Autodesk Inventor part; units mm, degrees
ref_plane "YZ Plane" through (0, 0, 0) normal (1, 0, 0) x (0, 1, 0)
ref_plane "XZ Plane" through (0, 0, 0) normal (0, 1, 0) x (-1, 0, 0)
ref_plane "XY Plane" through (0, 0, 0) normal (0, 0, 1) x (1, 0, 0)
sketch "Sketch1" plane through (0, 0, 0) normal (0, 1, 0) x (-1, 0, 0)
  line L0 (0, 0) -> (25.4, 0)
  line L1 (25.4, 0) -> (25.4, -127)
  line L2 (25.4, -127) -> (0, -127)
  line L3 (0, -127) -> (0, 0)
  line L4 (30.48, 5.08) -> (-5.08, 5.08)
  line L5 (-5.08, 5.08) -> (-5.08, -132.08)
  line L6 (-5.08, -132.08) -> (30.48, -132.08)
  line L7 (30.48, -132.08) -> (30.48, 5.08)
  dimension "d0" = 25.4
  dimension "d1" = 127
  dimension "d2" = 5.08
  dimension "d3" = 5.08
  dimension "d4" = 5.08
  dimension "d5" = 5.08
extrude "Extrusion1" add sketch "Sketch1" along normal blind 38.1
sketch "Sketch2" plane through (0, 38.1, 0) normal (0, 1, 0) x (1, 0, 0)
  line L0 (-30.48, -5.08) -> (5.08, -5.08)
  line L1 (5.08, -5.08) -> (-62.5812, -5.08)
  line L2 (-62.5812, -5.08) -> (-62.5812, 0)
  line L3 (-62.5812, 0) -> (0, 0)
  line L4 (-25.4, 127) -> (0, 127)
  line L5 (0, 127) -> (-62.5812, 127)
  line L6 (5.08, -5.08) -> (5.08, 132.08)
  line L7 (5.08, -5.08) -> (-62.5812, -5.08)
  line L8 (-62.5812, 132.08) -> (5.08, 132.08)
  line L9 (5.08, 132.08) -> (5.08, -5.08)
  line L10 (-62.5812, 132.08) -> (-47.0844, 132.08)
  line L11 (-62.5812, 127) -> (-62.5812, 132.08)
  line L12 (0, 127) -> (0, 0)
  line L13 (0, 0) -> (0, 127)
  line L14 (0, 127) -> (-62.5812, 127)
  line L15 (-62.5812, 132.08) -> (3.2473, 132.08)
  line L16 (5.08, 132.08) -> (-30.48, 132.08)
extrude "Extrusion2" add sketch "Sketch2" along normal blind 25.4
sketch "Sketch5" plane through (0, 38.1, 0) normal (0, -1, 0) x (1, 0, 0)
  line L0 (-62.5812, -132.08) -> (-62.5812, -127)
  line L1 (-30.48, -132.08) -> (-30.48, 5.08)
  line L2 (-62.5812, -132.08) -> (-30.48, -132.08)
  line L3 (-30.48, -132.08) -> (-30.48, -126.7104)
  line L4 (-30.48, -126.7104) -> (-62.5812, -126.7104)
  line L5 (-62.5812, -126.7104) -> (-62.5812, -132.08)
  line L6 (-62.5812, 0) -> (-62.5812, 5.08)
  line L7 (-30.48, 5.08) -> (5.08, 5.08)
  line L8 (-62.5812, 0) -> (-30.48, 0)
  line L9 (-30.48, 0) -> (-30.48, 5.08)
  line L10 (-30.48, 5.08) -> (-62.5812, 5.08)
  line L11 (-62.5812, 5.08) -> (-62.5812, 0)
  point P0 (0, 0)
extrude "Extrusion3" add sketch "Sketch5" along normal blind 38.1
sketch "Sketch6" plane through (-30.48, 0, 0) normal (-1, 0, 0) x (0, 0, 1)
  line L0 (-25.4, 7.62) -> (-38.1, 7.62)
  line L1 (-38.1, 7.62) -> (-38.1, 29.972)
  line L2 (-38.1, 29.972) -> (-25.4, 29.972)
  line L3 (-25.4, 29.972) -> (-25.4, 7.62)
  line L4 (-126.7104, 0) -> (0, 0)
  line L5 (0, 63.5) -> (0, 0)
  line L6 (-88.6104, 7.62) -> (-101.3104, 7.62)
  line L7 (-101.3104, 7.62) -> (-101.3104, 29.972)
  line L8 (-101.3104, 29.972) -> (-88.6104, 29.972)
  line L9 (-88.6104, 29.972) -> (-88.6104, 7.62)
  line L10 (-126.7104, 38.1) -> (-126.7104, 0)
  point P0 (-25.4, 18.796)
  point P1 (-88.6104, 18.796)
  point P2 (-126.7104, 19.05)
  point P3 (-101.3104, 18.796)
  dimension "d12" = 12.7
  dimension "d13" = 22.352
  dimension "d14" = 7.62
  dimension "d15" = 25.4
  dimension "d16" = 12.7
  dimension "d17" = 22.352
  dimension "d18" = 25.4
  dimension "d19" = 7.62
extrude "Extrusion4" cut sketch "Sketch6" against normal blind 12.7
sketch "Sketch7" plane through (0, 0, -127) normal (-1, 0, 0) x (0, 0, 1)
  line L0 (51.0896, 34.798) -> (38.3896, 34.798)
  line L1 (38.3896, 34.798) -> (38.3896, 57.15)
  line L2 (38.3896, 57.15) -> (51.0896, 57.15)
  line L3 (51.0896, 57.15) -> (51.0896, 34.798)
  line L4 (38.3896, 29.972) -> (38.3896, 7.62)
  line L5 (0, 63.5) -> (127, 63.5)
  line L6 (114.3, 34.798) -> (101.6, 34.798)
  line L7 (101.6, 34.798) -> (101.6, 57.15)
  line L8 (101.6, 57.15) -> (114.3, 57.15)
  line L9 (114.3, 57.15) -> (114.3, 34.798)
  line L10 (101.6, 31.5595) -> (101.6, 9.2075)
  line L11 (101.6, 29.972) -> (101.6, 7.62)
  point P0 (127, 0)
  point P1 (51.0896, 45.974)
  point P2 (38.3896, 18.796)
  point P3 (44.7396, 57.15)
  point P4 (114.3, 45.974)
  point P5 (101.6, 20.3835)
  point P6 (107.95, 57.15)
  dimension "d22" = 12.7
  dimension "d23" = 22.352
  dimension "d24" = 0
  dimension "d25" = 6.35
  dimension "d26" = 12.7
  dimension "d27" = 22.352
  dimension "d28" = 0
  dimension "d29" = 6.35
extrude "Extrusion5" cut sketch "Sketch7" against normal blind 12.7
properties part number "Base1"
Geometry check sheet. Reference: the model listing, model coordinates, mm. A direction names the side the tool comes from. Coordinates: 2 decimals unless noted, no trailing zeros. Order: outer loops, then holes, each group sorted by start corner. A loop starts at its lowest first (then second) coordinate and runs counter-clockwise, first axis right, second up. Notation, with made-up numbers: (-26.5, -37) - (4.5, -37) arc R12 cw to (4.5, -32) - close; hole circle Ø7 at (-31.75, 55.25). An arc over 180 degrees is marked (long way). Answer as a JSON object with one key per item and string values. Group by question number.
Item 1: Sectioned sample at C-C, the plane z = -86. Record the cut outline in (x, y), and give its area (3 significant figures).
Item 2: Draft check along Z on faces 1 (the face through (-29, 31, 5.08)), 2 (the face through (3, 57.15, -82)), 3 (the face through (5.08, 31, -63)). Enter one of: +Z half, -Z half, draft (parallel to the pull), parting line (faces both ways), or undercut.
Item 3: Scan lines: probe 1 along Z at (x, y) = (-8.5, 53.5); probe 2 along Z at (x, y) = (-58.5, 6); probe 3 along X at (y, z) = (6.5, -35). Record each from-to range of solid material in increasing order.
Item 4: Sectioned sample at B-B, the plane x = -5. Record the cut outline in (y, z).
Item 5: Sectioned sample at A-A, the plane y = 39.5. Record the cut outline in (x, z).
Item 6: Sectioned sample at D-D, the plane y = 13. Record the cut outline in (x, z), and give its area (3 significant figures).
Item 7: Depth check by flat-ended pin: pin 1 Ø19 at (y, z) = (21.5, -47.5) entering from -X; pin 2 Ø3 at (y, z) = (40.5, -12) entering from -X; pin 3 Ø2.5 at (x, z) = (-28.5, -96) entering from +Y. Enter the tip coordinate at first touch or a pass-through.
Item 8: Tool access check on faces 4 (the face through (-30.48, 19, -64)), 5 (the face through (3, 34.798, -19)), 6 (the face through (-28, 7.62, -32)), 7 (the face through (3, 57.15, -19)), 8 (the face through (-25.4, 19, -63)). Record the directions out of +Z, -Z, +X, -X, +Y, -Y that give a thin tool (end or side, any length) a straight path to the whole face; none if there is none.
Resolved:
{
 "1": {"outline": "(-30.48, 0) - (-25.4, 0) - (-25.4, 38.1) - (-30.48, 38.1) - close; (0, 0) - (5.08, 0) - (5.08, 34.8) - (0, 34.8) - close; (0, 57.15) - (5.08, 57.15) - (5.08, 63.5) - (0, 63.5) - close", "area": "403 mm^2"},
 "2": {"face 1": "+Z half", "face 2": "undercut", "face 3": "draft"},
 "3": {"probe 1": "-132.08 to -127, 0 to 5.08", "probe 2": "-132.08 to -126.71, 0 to 5.08", "probe 3": "-30.48 to -25.4, 0 to 5.08"},
 "4": {"outline": "(0, -132.08) - (63.5, -132.08) - (63.5, -127) - (0, -127) - close; (0, 0) - (63.5, 0) - (63.5, 5.08) - (0, 5.08) - close"},
 "5": {"outline": "(-62.58, -132.08) - (5.08, -132.08) - (5.08, -88.61) - (0, -88.61) - (0, -127) - (-62.58, -127) - close; (-62.58, 0) - (0, 0) - (0, -12.7) - (5.08, -12.7) - (5.08, 5.08) - (-62.58, 5.08) - close; (0, -75.91) - (5.08, -75.91) - (5.08, -25.4) - (0, -25.4) - close"},
 "6": {"outline": "(-62.58, -132.08) - (5.08, -132.08) - (5.08, 5.08) - (-62.58, 5.08) - (-62.58, 0) - (-30.48, 0) - (-30.48, -25.4) - (-25.4, -25.4) - (-25.4, 0) - (0, 0) - (0, -127) - (-25.4, -127) - (-25.4, -101.31) - (-30.48, -101.31) - (-30.48, -126.71) - (-62.58, -126.71) - close; (-30.48, -88.61) - (-25.4, -88.61) - (-25.4, -38.1) - (-30.48, -38.1) - close", "area": "1,860 mm^2"},
 "7": {"pin 1": "x = -30.48", "pin 2": "x = 0", "pin 3": "y = 38.1"},
 "8": {"face 4": "-X, +Y, -Y", "face 5": "+X", "face 6": "-X", "face 7": "+X, -X", "face 8": "+Y, -Y"}
}
